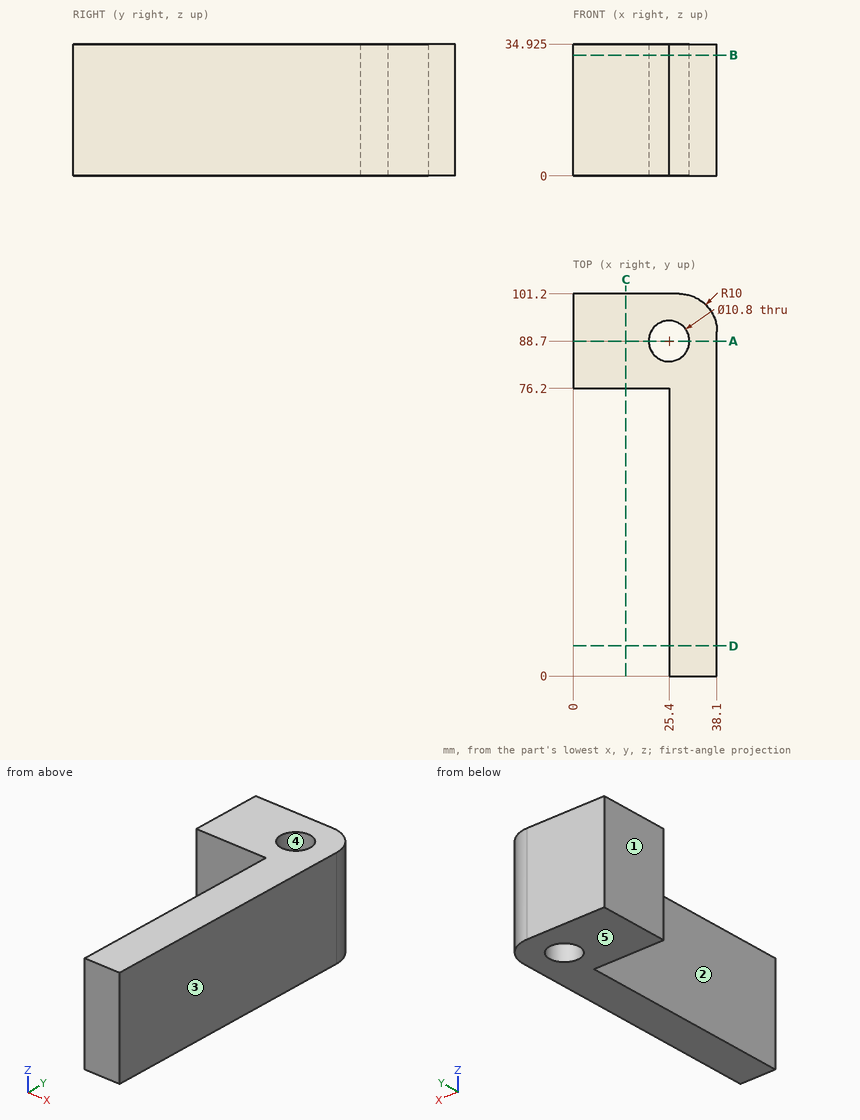
Could you check a few things on this drawing? It's one solid part, dimensions in mm from its lowest x, y, z. A direction names the side the tool comes from. Round coordinates to 2 decimals unless told otherwise and drop trailing zeros. Write each loop counter-clockwise with the first axis right and the second up, starting at its lowest first coordinate (ties: lowest second). Pieces come first, ordered by that corner, then holes.
Q1. If we section it at A-A on y = 88.7: Write out the boundary of the cut face in (x, z) (3 decimals).
Q2. If we section it at C-C on x = 14: Write out the boundary of the cut face in (y, z) (3 decimals), plus the area to 3 significant figures.
Q3. If we section it at B-B on z = 32: Write out the boundary of the cut face in (x, y), plus the area to 3 significant figures.
Q4. Will these pins go through, and if not, where does the flat tip stop? P1, Ø20.5, axis at x = 10.5, z = 13, coming from the -Y side; P2, Ø5, axis at y = 86, z = 3.5, coming from the -X side; P3, Ø17.5, axis at y = 26.5, z = 17.5, coming from the -X side.
Q5. Please list where these lines run through material, in increasing order: probe 1 along Y at (x, z) = (25, 18); probe 2 along X at (y, z) = (15.5, 28.5); probe 3 along Y at (x, z) = (18, 20).
Q6. If we section it at D-D on y = 8: Write out the boundary of the cut face in (x, z) (3 decimals).
Q7. If we mould it in two halves opening along X, with no side actions, what happens to the marked faces 3, 4 and 5? For each: +X half, -X half, draft (parallel to the pull), parting line (faces both ways), or undercut.
Q8. Which directions (+Z, -Z, +X, -X, +Y, -Y) give clear straight access to the entire face, cutting with the end or side of a thin tool? Please do the marked faces 1 and 2.
Answer below:
1. outline: (0, 0) - (20, 0) - (20, 34.925) - (0, 34.925) - close; (30.8, 0) - (38.1, 0) - (38.1, 34.925) - (30.8, 34.925) - close
2. outline: (76.2, 0) - (101.2, 0) - (101.2, 34.925) - (76.2, 34.925) - close
2. area: 873 mm2
3. outline: (0, 76.2) - (25.4, 76.2) - (25.4, 0) - (38.1, 0) - (38.1, 91.2) arc R10 ccw to (28.1, 101.2) - (0, 101.2) - close; hole circle Ø10.8 at (25.4, 88.7)
3. area: 1,810 mm2
4. P1: stops at y = 76.2
4. P2: stops at x = 0
4. P3: stops at x = 25.4
5. probe 1: y = 76.2 to 83.31, 94.09 to 101.2
5. probe 2: x = 25.4 to 38.1
5. probe 3: y = 76.2 to 101.2
6. outline: (25.4, 0) - (38.1, 0) - (38.1, 34.925) - (25.4, 34.925) - close
7. face 3: +X half
7. face 4: undercut
7. face 5: draft
8. face 1: +Z, -Z, -X, +Y, -Y
8. face 2: +Z, -Z, -X, -Y
